The listing builds one solid part. Answer for the finished solid, in the listing's coordinates (mm). A direction names the side the tool comes from. Give positions to 0.01 mm unless a question says otherwise; leave off trailing zeros. Loops run counter-clockwise (first coordinate to the right, second up) from the corner with the lowest first, then second, coordinate; pieces in that order, holes last. Notation, with made-up numbers: (-19, 8) -> (9, 8) arc R18 cw to (9, 20) -> close; hole circle Ø3 at (-29, 56.25). An arc over 180 degrees is marked (long way). One line per question, with ' | ' between items. Start each with the question number.
Autodesk Inventor part; units mm, degrees
ref_plane "YZ Plane" through (0, 0, 0) normal (1, 0, 0) x (0, 1, 0)
ref_plane "XZ Plane" through (0, 0, 0) normal (0, 1, 0) x (-1, 0, 0)
ref_plane "XY Plane" through (0, 0, 0) normal (0, 0, 1) x (1, 0, 0)
sketch "Sketch1" plane through (0, 0, 0) normal (0, 1, 0) x (-1, 0, 0)
  line L0 (0, 0) -> (10, 0)
  line L1 (10, 0) -> (10, 20)
  line L2 (10, 20) -> (0, 20)
  line L3 (0, 20) -> (0, 0)
  dimension "d0" = 10
  dimension "d1" = 20
extrude "Extrusion1" add sketch "Sketch1" along normal blind 5
sketch "Sketch2" plane through (0, 5, 0) normal (0, 1, 0) x (1, 0, 0)
  line L0 (-10, -20) -> (0, -20)
  line L1 (-6.9999, -20) -> (-2.9999, -20)
  line L2 (-2.9999, -20) -> (-2.9999, -17)
  line L3 (-2.9999, -17) -> (-6.9999, -17)
  line L4 (-6.9999, -17) -> (-6.9999, -20)
  point P0 (0, 0)
  dimension "d4" = 4
  dimension "d5" = 3
extrude "Extrusion2" add sketch "Sketch2" along normal blind 5
sketch "Sketch3" plane through (0, 5, 0) normal (0, 1, 0) x (1, 0, 0)
  line L0 (-10.0114, 0) -> (-0.0114, 0)
  line L1 (-0.0114, 0) -> (-0.0114, -3)
  line L2 (-0.0114, -3) -> (-10.0114, -3)
  line L3 (-10.0114, -3) -> (-10.0114, 0)
  point P0 (0, 0)
  dimension "d8" = 10
  dimension "d9" = 3
extrude "Extrusion3" add sketch "Sketch3" along normal blind 5
sketch "Sketch4" plane through (-10, 0, 20) normal (0, 0, 1) x (1, 0, 0)
  circle A0 centre (5.0001, 9) radius 1
  point P0 (10, 0)
  dimension "d12" = 2
extrude "Extrusion4" cut sketch "Sketch4" against normal blind 21.9875
sketch "Sketch5" plane through (-10, 0, 20) normal (0, 0, 1) x (1, 0, 0)
  circle A0 centre (5.0001, 9) radius 1
  line L0 (4.0001, 9) -> (6.0001, 9)
  line L1 (6.0001, 9) -> (6.0001, 10)
  line L2 (6.0001, 10) -> (4.0001, 10)
  line L3 (4.0001, 10) -> (4.0001, 9)
  point P0 (10, 0)
  dimension "d15" = 2
  dimension "d16" = 1
extrude "Extrusion5" cut sketch "Sketch5" against normal blind 22.4625 contours L3 L2 A0 | A0 L0 | A0 L2 L1 picked at (5.3251, 9.0742)
sketch "Sketch6" plane through (-10, 0, 20) normal (0, 0, 1) x (1, 0, 0)
  arc A0 (4.0001, 9) -> (6.0001, 9) centre (5.0001, 9) ccw
  line L0 (4.0001, 9) -> (6.0001, 9)
  line L1 (6.0001, 9) -> (6.0001, 10.3931)
  line L2 (6.0001, 10.3931) -> (4.0001, 10.3931)
  line L3 (4.0001, 10.3931) -> (4.0001, 9)
  point P0 (10, 0)
extrude "Extrusion6" cut sketch "Sketch6" against normal blind 25.1625 contours L3 L2 L1 L0
sketch "Sketch7" plane through (0, 5, 0) normal (0, 1, 0) x (1, 0, 0)
  point P0 (0, 0)
sketch "Sketch8" plane through (0, 0, 0) normal (0, 0, -1) x (-1, 0, 0)
  point P0 (0, 0)
equation "\"BendRadius\" = Thickness"
equation "\"BendReliefWidth\" = Thickness"
equation "\"BendReliefDepth\" = 0.5 * Thickness"
equation "\"CornerReliefSize\" = 4 * Thickness"
equation "\"MinimumRemnant\" = 2 * Thickness"
equation "\"TransitionRadius\" = BendRadius"
equation "\"JacobiRadiusSize\" = BendRadius"
equation "\"GapSize\" = Thickness"
properties part number "uchwyt_swiatlowod_2"
1. Determine the mould class of faces 6 (the flat face through (-2, 10, 1)), 7 (the flat face through (-0.011, 7, 1)), 8 (the flat face through (-6, 9.5, 1.5)) for opening direction X: released by +X, released by -X, zero draft, split by the parting line, or undercut.
2. The part is cut by section D-D (x = -1). Write down the section's boundary in (y, z), plus the area to 3 significant figures.
3. Each of these flat-tipped pins is pushed along its axis until it touches: pin 1 Ø1.1 at (y, z) = (9.5, 18) entering from +X; pin 2 Ø3 at (x, z) = (-2.5, 5.5) entering from +Y; pin 3 Ø2.5 at (y, z) = (3, 6) entering from -X. Where does it stop, or does it pass through?
4. The part is cut by section A-A (y = 6.5). Write down the section's boundary in (x, z), plus the area to 3 significant figures.
5. For faces 1 (the flat face through (-4, 9.5, 1.5)), 2 (the flat face through (-6.5, 10, 18.5)), 3 (the flat face through (-3, 7, 19)), 4 (the flat face through (-5, 7, 17)), 5 (the flat face through (-5, 4, 20)), determine the directions among +Z, -Z, +X, -X, +Y, -Y from which every point of the face is accessible in a straight line to the end or side of a thin tool.
6. The part is cut by section B-B (x = -3.25). Write down the section's boundary in (y, z), plus the area to 3 significant figures.
7. Straight lines are drawn through the part: L1, parallel to Z at x = -4.5, y = 6.75; L2, parallel to X at y = 9.25, z = 2.25; L3, parallel to X at y = 3.25, z = 17. For each, find the intervals that lie inside material, in ascending order.
Check sheet entries:
1) face 6: zero draft | face 7: released by +X | face 8: undercut
2) outline: (0, 0) -> (10, 0) -> (10, 3) -> (5, 3) -> (5, 20) -> (0, 20) -> close | area: 115 mm^2
3) pin 1: stops at x = -3 | pin 2: stops at y = 5 | pin 3: stops at x = -10
4) outline: (-10.01, 0) -> (-0.01, 0) -> (-0.01, 3) -> (-10.01, 3) -> close; (-7, 17) -> (-3, 17) -> (-3, 20) -> (-7, 20) -> close | area: 42.0 mm^2
5) face 1: +Z, -Z, +Y | face 2: +Z, -Z, +X, -X, +Y | face 3: +Z, +X, +Y | face 4: +X, -X, +Y | face 5: +Z, +X, -X, +Y, -Y
6) outline: (0, 0) -> (10, 0) -> (10, 3) -> (5, 3) -> (5, 17) -> (10, 17) -> (10, 20) -> (0, 20) -> close | area: 130 mm^2
7) L1: z = 0 to 3, 17 to 20 | L2: x = -10.01 to -6, -4 to -0.01 | L3: x = -10 to 0
